Here's how the part is built. I have some questions about the finished solid (model axes, mm). A direction names the side the tool comes from. Round coordinates to 2 decimals unless told otherwise and drop trailing zeros. Write each loop counter-clockwise with the first axis right and the second up, starting at its lowest first coordinate (ties: lowest second). Pieces come first, ordered by that corner, then holes. Notation, with made-up numbers: (-22.5, 85.5) -> (18.5, 85.5) arc R32 ccw to (18.5, 113.5) -> close; hole circle Ø2 at (71.5, 54). An arc over 180 degrees is marked (long way). Answer as CSV lines item,"result".
from build123d import *

# Parameters (mm, degrees)
F1_DEPTH    = 25
F2_T4_DEPTH = 25
F3_R        = 2
F4_R        = 1
F5_R        = 5
F6_R        = 2
F8_DEPTH    = 25.001
F9_R        = 3


# Not quite as in the source:
# - a fillet or chamfer that OpenCascade refuses, or shapes differently, is made with other operations: its cross-section is extruded or revolved along the edge and cut away or added


with BuildPart() as f1:
    # F0 (on Top) → F1 (new body)
    with BuildSketch(Plane.XY):
        with BuildLine():
            ThreePointArc((11.3, -11.9364390799), (9.4662629179, -9.9817974282), (7.3, -8.4036590808))
            Line((7.3, -8.4036590808), (7.3, -12.0744565389))
            ThreePointArc((7.3, -12.0744565389), (10.2513413756, -15.9460542704), (11.3, -20.7))
            Line((11.3, -20.7), (11.3, -11.9364390799))
        make_face()
        with BuildLine():
            ThreePointArc((11.3, 11.9364390799), (9.4662629179, 9.9817974282), (7.3, 8.4036590808))
            Line((7.3, 8.4036590808), (7.3, -8.4036590808))
            ThreePointArc((7.3, -8.4036590808), (9.4662629179, -9.9817974282), (11.3, -11.9364390799))
            Line((11.3, -11.9364390799), (11.3, -2))
            Line((11.3, -2), (11.3, 2))
            Line((11.3, 2), (11.3, 11.9364390799))
        make_face()
        with BuildLine():
            ThreePointArc((11.3, 20.7), (10.2513413756, 15.9460542704), (7.3, 12.0744565389))
            Line((7.3, 12.0744565389), (7.3, 8.4036590808))
            ThreePointArc((7.3, 8.4036590808), (9.4662629179, 9.9817974282), (11.3, 11.9364390799))
            Line((11.3, 11.9364390799), (11.3, 20.7))
        make_face()
        with BuildLine():
            ThreePointArc((-7.9903066274, 28.6903066274), (4.3243227857, 31.1398387174), (11.3, 20.7))
            Line((11.3, 20.7), (11.3, 11.9364390799))
            ThreePointArc((11.3, 11.9364390799), (13.5292276202, 16.0685855292), (14.3, 20.7))
            ThreePointArc((14.3, 20.7), (5.4723730828, 33.9114773149), (-10.111626971, 30.811626971))
            Line((-10.111626971, 30.811626971), (-7.9903066274, 28.6903066274))
        make_face()
        with BuildLine():
            Line((7.3, 8.4036590808), (7.3, 12.0744565389))
            ThreePointArc((7.3, 12.0744565389), (-0.4690546543, 9.4097392532), (-7.9903066274, 12.7096933726))
            Line((-7.9903066274, 12.7096933726), (-10.111626971, 10.588373029))
            ThreePointArc((-10.111626971, 10.588373029), (-1.7803244971, 6.5112564092), (7.3, 8.4036590808))
        make_face()
        with BuildLine():
            Line((7.3, -12.0744565389), (7.3, -8.4036590808))
            ThreePointArc((7.3, -8.4036590808), (-1.7803244971, -6.5112564092), (-10.111626971, -10.588373029))
            Line((-10.111626971, -10.588373029), (-7.9903066274, -12.7096933726))
            ThreePointArc((-7.9903066274, -12.7096933726), (-0.4690546543, -9.4097392532), (7.3, -12.0744565389))
        make_face()
        with BuildLine():
            ThreePointArc((14.3, -20.7), (13.5292276202, -16.0685855292), (11.3, -11.9364390799))
            Line((11.3, -11.9364390799), (11.3, -20.7))
            ThreePointArc((11.3, -20.7), (4.3243227857, -31.1398387174), (-7.9903066274, -28.6903066274))
            Line((-7.9903066274, -28.6903066274), (-10.111626971, -30.811626971))
            ThreePointArc((-10.111626971, -30.811626971), (5.4723730828, -33.9114773149), (14.3, -20.7))
        make_face()
        Polygon((27.3, 2), (11.3, 2), (11.3, -2), (31.3, -2), (31.3, 13), (27.3, 13), align=None)
    extrude(amount=F1_DEPTH)

    # F2: chamfer of 20 on 1 edges, made by hand


with BuildPart() as f2_tool2:
    # F2_s3 → F2_t4 (new body)
    with BuildSketch(Plane.XY):
        Polygon((11.3, -22), (31.3, -2), (11.3, -2), align=None)
    extrude(amount=F2_T4_DEPTH)

    split(bisect_by=Plane.YZ.offset(31.3), keep=Keep.BOTTOM)


with BuildPart() as f1_1:
    add(f1.part)

    # F2_t1: union F2_tool2
    add(f2_tool2.part)

    # F3
    f3_edges = [f1_1.edges().sort_by_distance(p)[0] for p in [
        (27.3, 2, 12.5),
        (11.3, 2, 12.5),
    ]]
    fillet(f3_edges, radius=F3_R)

    # F4
    f4_edges = [f1_1.edges().sort_by_distance(p)[0] for p in [
        (31.3, 13, 12.5),
        (27.3, 13, 12.5),
        (-7.990307, -12.709693, 12.5),
        (-10.111627, -10.588373, 12.5),
        (-7.990307, -28.690307, 12.5),
        (-10.111627, -30.811627, 12.5),
        (-10.111627, 10.588373, 12.5),
        (-7.990307, 12.709693, 12.5),
        (-7.990307, 28.690307, 12.5),
        (-10.111627, 30.811627, 12.5),
    ]]
    fillet(f4_edges, radius=F4_R)

    # F5
    f5_edges = [f1_1.edges().sort_by_distance(p)[0] for p in [
        (11.3, 11.936439, 12.5),
        (31.3, -2, 12.5),
        (14.209172, -19.090828, 12.5),
    ]]
    fillet(f5_edges, radius=F5_R)

    # F6
    f6_edges = [f1_1.edges().sort_by_distance(p)[0] for p in [
        (7.3, 8.403659, 12.5),
        (7.3, -8.403659, 12.5),
    ]]
    fillet(f6_edges, radius=F6_R)

    # F7 (on face) → F8 (cut, through all)
    with BuildSketch(Plane.XY.offset(25)):
        Polygon((28.0573593129, -1), (11.3, -1), (11.3, -17.7573593129), align=None)
    extrude(amount=-F8_DEPTH, mode=Mode.SUBTRACT)

    # F9
    f9_edges = [f1_1.edges().sort_by_distance(p)[0] for p in [
        (11.3, -1, 12.5),
        (28.057359, -1, 12.5),
        (11.3, -17.757359, 12.5),
    ]]
    fillet(f9_edges, radius=F9_R)


solid = f1_1.part
Item 1: Will these pins go through, and if not, where does the flat tip stop? pin 1 (7 mm diameter, centred on y = -6.5, z = 15.5, fed in from +X); pin 2 (0.6 mm diameter, centred on x = 29, z = 11.5, fed in from +Y); pin 3 (3 mm diameter, centred on y = -7.5, z = 15.5, fed in from -X); pin 4 (9 mm diameter, centred on y = 7, z = 7.5, fed in from -X).
Results found:
pin 1,"stops at x = 30.25"
pin 2,"stops at y = 13"
pin 3,"stops at x = -8.22"
pin 4,"stops at x = -9.67"
Item 2: Suppose I cut it at B-B, the plane x = -3.5. List the corners of the cut face in (y, z) for me.
Results found:
outline,"(-34.57, 0) -> (-31.44, 0) -> (-31.44, 25) -> (-34.57, 25) -> close; (-9.96, 0) -> (-6.83, 0) -> (-6.83, 25) -> (-9.96, 25) -> close; (6.83, 0) -> (9.96, 0) -> (9.96, 25) -> (6.83, 25) -> close; (31.44, 0) -> (34.57, 0) -> (34.57, 25) -> (31.44, 25) -> close"
Item 3: Suppose I cut it at A-A, the plane x = 17.5. List the corners of the cut face in (y, z) for me, then the cut area to 3 significant figures.
Results found:
outline,"(-15.8, 0) -> (-11.56, 0) -> (-11.56, 25) -> (-15.8, 25) -> close; (-1, 0) -> (2, 0) -> (2, 25) -> (-1, 25) -> close"
area,"181 mm²"
Item 4: If we mould it in two halves opening along Y, with no side actions, what happens to faces 1 (the cylindrical face through (-2.796, 6.676, 12.325)), 2 (the flat face through (27.3, 8, 12)), 3 (the cylindrical face through (5.632, -33.844, 12.325))? For each: pulls with the +Y half, pulls with the -Y half, needs draft (parallel to the pull), parting line crosses it, or undercut.
Results found:
face 1,"undercut"
face 2,"needs draft"
face 3,"pulls with the -Y half"
Item 5: I need wall thicknesses on L1, parallel to Y at x = 8, z = 14.75; L2, parallel to Y at x = 7.5, z = 4.5; L3, parallel to Y at x = -2.5, z = 11.5. Which ranges of each line are inside material? Lowest first, please.
Results found:
L1,"y = -32.55 to -28.68, -12.72 to 12.72, 28.68 to 32.55"
L2,"y = -32.88 to -29.15, -12.25 to 12.25, 29.15 to 32.88"
L3,"y = -34.78 to -31.72, -9.68 to -6.62, 6.62 to 9.68, 31.72 to 34.78"
Item 6: Suppose I cut it at D-D, the plane y = -26. List the corners of the cut face in (x, z) for me, then the cut area to 3 significant figures.
Results found:
outline,"(9.98, 0) -> (13.28, 0) -> (13.28, 25) -> (9.98, 25) -> close"
area,"82.5 mm²"
Item 7: For faces 4 (the cylindrical face through (12.2, -1.86, 12.32)), 5 (the flat face through (7.3, 0, 12)), 6 (the flat face through (29, 13, 12)), which set-ups out of +Z, -Z, +X, -X, +Y, -Y let a thin tool reach every point of the face, with its end or its side?
Results found:
face 4,"+Z, -Z"
face 5,"+Z, -Z, -X"
face 6,"+Z, -Z, +X, +Y"
Item 8: Suppose I cut it at C-C, the plane x = 9. List the corners of the cut face in (y, z) for me, then the cut area to 3 significant figures.
Results found:
outline,"(-31.81, 0) -> (-27.53, 0) -> (-27.53, 25) -> (-31.81, 25) -> close; (-13.87, 0) -> (13.87, 0) -> (13.87, 25) -> (-13.87, 25) -> close; (27.53, 0) -> (31.81, 0) -> (31.81, 25) -> (27.53, 25) -> close"
area,"907 mm²"
